Check sheet for the modelled part. Datum: model origin and axes. Units: mm. A direction names the side the tool comes from. Give positions to 0.01 mm unless a question says otherwise; leave off trailing zeros. Order: outer loops, then holes, each group sorted by start corner. A loop starts at its lowest first (then second) coordinate and runs counter-clockwise, first axis right, second up. Notation, with made-up numbers: (29, 34.25) -> (46, 34.25) arc R17 cw to (46, 56.25) -> close; hole circle Ø5 at (-28, 49). An arc over 180 degrees is marked (long way). Answer in a Markdown table with one row per item. Add a question column.
(1) Cross-section at A-A (y = -34). Record the cut outline in (x, z).
(2) Release check for a two-part mould opening along X. For faces 4 (the face through (9.26, -2.32, 11.39)), 5 (the face through (10.8, -18, 8)), 6 (the face through (1.6, -2, 6.6)) record: released by +X, released by -X, zero draft, split by the parting line, or undercut.
(3) Set-up check for faces 1 (the face through (1.3, -6, 7.6)), 2 (the face through (0, -2, 11)), 3 (the face through (0, -37, 8)): record each of +Z, -Z, +X, -X, +Y, -Y from which the full face is reachable in a straight line by a thin tool's end or side.
(4) Cross-section at C-C (z = 13.5). Record the cut outline in (x, y).
(5) Go/stop test with flat-tipped pins: pin 1 (1.3 mm diameter, centred on y = -2.7, z = 10.8, fed in from +X); pin 2 (2 mm diameter, centred on y = -2.7, z = 10.8, fed in from -X). Record where each tip stops, or that it passes through.
(6) Cross-section at D-D (x = 0). Record the cut outline in (y, z).
(7) Cross-section at B-B (y = -2.7). Record the cut outline in (x, z), then the cut area to 3 significant figures.
(8) Thickness scan on L1, parallel to Y at x = 8.8, z = 10.8; L2, parallel to Z at x = 9.95, y = -34; L3, parallel to Z at x = -3.95, y = -2.7. Record the ranges inside material, lowest first. Write a range as [from, to].
```python
from build123d import *

# Parameters (mm, degrees)
PAD_DEPTH         = 35
SKETCH001_W       = 21.6
SKETCH001_H       = 15.8
PAD001_DEPTH      = 2
SKETCH002_R       = 4.3
SKETCH002_R_2     = 3.3
PAD002_DEPTH      = 6
SKETCH003_R       = 0.7
POCKET_DEPTH      = 10.801
POCKET_DEPTH_BACK = 10.801
SKETCH004_W       = 21.6
SKETCH004_H       = 15.8
PAD003_DEPTH      = 2


with BuildPart() as part:
    # Sketch → Pad (new body)
    with BuildSketch(Plane.XZ):
        with BuildLine():
            Line((-10.8, 0), (10.8, 0))
            Line((10.8, 0), (10.8, 15.8))
            Line((10.8, 15.8), (7.8, 15.8))
            Line((7.8, 15.8), (7.8, 10.8))
            ThreePointArc((-7.8, 10.8), (0, 3), (7.8, 10.8))
            Line((-7.8, 10.8), (-7.8, 15.8))
            Line((-7.8, 15.8), (-10.8, 15.8))
            Line((-10.8, 15.8), (-10.8, 0))
        make_face()
    extrude(amount=PAD_DEPTH)

    # Sketch001 → Pad001 (join)
    with BuildSketch(Plane.XZ):
        with Locations((0, 7.9)):
            Rectangle(SKETCH001_W, SKETCH001_H)
    extrude(amount=PAD001_DEPTH)

    # Sketch002 → Pad002 (join)
    with BuildSketch(Plane.XZ):
        with Locations((0, 10.8)):
            Circle(SKETCH002_R)
        with Locations((0, 10.8)):
            Circle(SKETCH002_R_2, mode=Mode.SUBTRACT)
    extrude(amount=PAD002_DEPTH)

    # Sketch003 → Pocket (cut, two sides)
    with BuildSketch(Plane.YZ) as pocket_sk:
        with Locations((-2.7, 10.8)):
            Circle(SKETCH003_R)
        with Locations((-34, 10.8)):
            Circle(SKETCH003_R)
    extrude(amount=-POCKET_DEPTH, mode=Mode.SUBTRACT)
    extrude(pocket_sk.sketch, amount=POCKET_DEPTH_BACK, mode=Mode.SUBTRACT)

    # Sketch004 (on DatumPlane) → Pad003 (join)
    with BuildSketch(Plane.XZ.offset(35)):
        with Locations((0, 7.9)):
            Rectangle(SKETCH004_W, SKETCH004_H)
    extrude(amount=PAD003_DEPTH)


solid = part.part
```
Answer below:
| question | item | result |
|---|---|---|
| 1 | outline | (-10.8, 0) -> (10.8, 0) -> (10.8, 10.1) -> (7.77, 10.1) arc R7.8 cw to (-7.77, 10.1) -> (-10.8, 10.1) -> close; (-10.8, 11.5) -> (-7.8, 11.5) -> (-7.8, 15.8) -> (-10.8, 15.8) -> close; (7.8, 11.5) -> (10.8, 11.5) -> (10.8, 15.8) -> (7.8, 15.8) -> close |
| 2 | face 4 | zero draft |
| 2 | face 5 | released by +X |
| 2 | face 6 | undercut |
| 3 | face 1 | +Z |
| 3 | face 2 | none |
| 3 | face 3 | +Z, -Z, +X, -X, -Y |
| 4 | outline | (-10.8, -37) -> (10.8, -37) -> (10.8, 0) -> (-10.8, 0) -> close; hole (-7.8, -35) -> (7.8, -35) -> (7.8, -2) -> (3.35, -2) -> (3.35, -6) -> (1.9, -6) -> (1.9, -2) -> (-1.9, -2) -> (-1.9, -6) -> (-3.35, -6) -> (-3.35, -2) -> (-7.8, -2) -> close |
| 5 | pin 1 | passes through |
| 5 | pin 2 | stops at x = -10.8 |
| 6 | outline | (-37, 0) -> (0, 0) -> (0, 15.8) -> (-2, 15.8) -> (-2, 15.1) -> (-6, 15.1) -> (-6, 14.1) -> (-2, 14.1) -> (-2, 7.5) -> (-6, 7.5) -> (-6, 6.5) -> (-2, 6.5) -> (-2, 3) -> (-35, 3) -> (-35, 15.8) -> (-37, 15.8) -> close |
| 7 | outline | (-10.8, 0) -> (10.8, 0) -> (10.8, 10.1) -> (7.77, 10.1) arc R7.8 cw to (-7.77, 10.1) -> (-10.8, 10.1) -> close; (-10.8, 11.5) -> (-7.8, 11.5) -> (-7.8, 15.8) -> (-10.8, 15.8) -> close; (-4.24, 10.1) arc R4.3 ccw to (4.24, 10.1) -> (3.22, 10.1) arc R3.3 cw to (-3.22, 10.1) -> close; (-4.24, 11.5) -> (-3.22, 11.5) arc R3.3 cw to (3.22, 11.5) -> (4.24, 11.5) arc R4.3 ccw to start; (7.8, 11.5) -> (10.8, 11.5) -> (10.8, 15.8) -> (7.8, 15.8) -> close |
| 7 | area | 180 mm² |
| 8 | L1 | y = [-37, -34.7], [-33.3, -3.4], [-2, 0] |
| 8 | L2 | z = [0, 10.1], [11.5, 15.8] |
| 8 | L3 | z = [0, 4.07], [9.1, 10.1], [11.5, 12.5] |
